Input: dimensioned drawing with shaded views. Units: mm. Origin: part minimum x, y, z. Give positions to 0.01 mm unless a question says otherwise; leave off trailing zeros. Loops run counter-clockwise (first coordinate to the right, second up) from the corner with the lowest first, then second, coordinate; pieces in that order, holes last. Notation, with made-up numbers: (-28, 18) -> (8, 18) arc R16 ccw to (8, 47) -> close; hole circle Ø3 at (57.5, 72). An arc over 180 degrees is marked (long way). Answer as a JSON object with one key per item and string values.
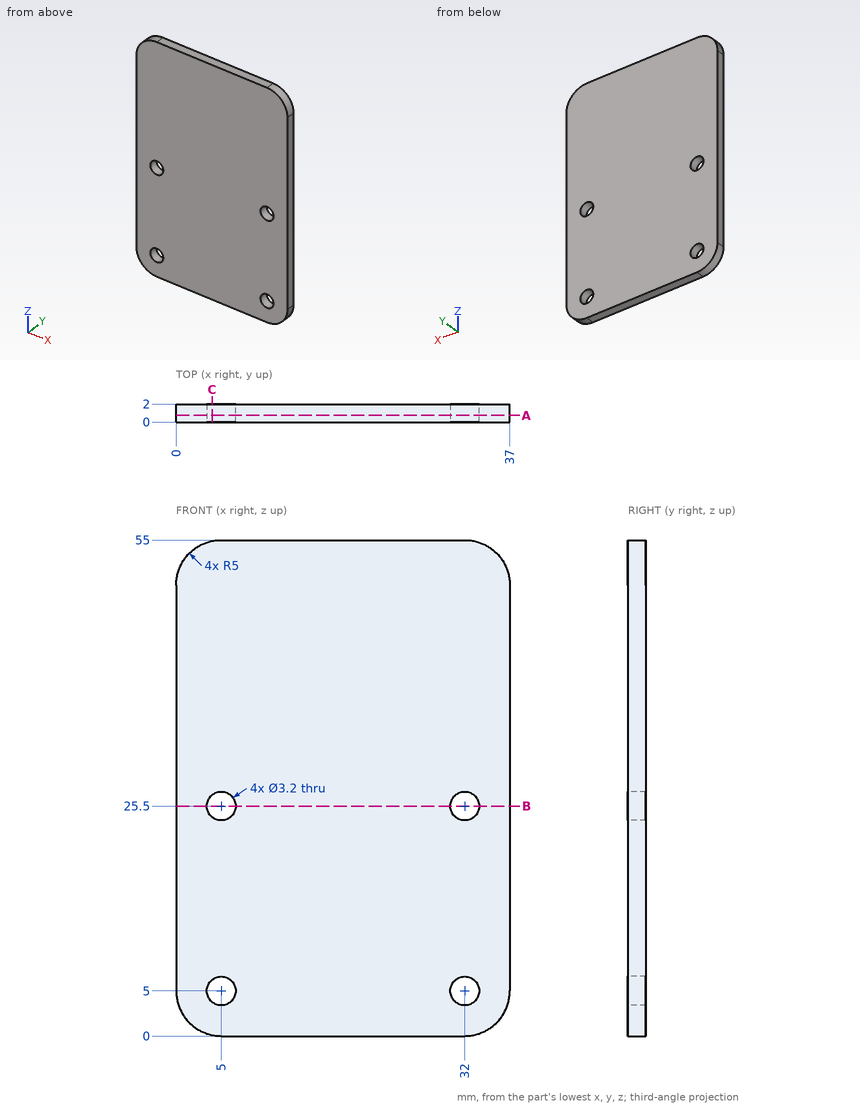
Q1. Ray query, line 1 along Z through (x, y) = (5, 0.8); line 2 along X through (y, z) = (0.9, 5); line 3 along X through (y, z) = (1.75, 4). Return the intervals inside material, ascending.
Evaluation:
{"line 1": "z = 0 to 3.4, 6.6 to 23.9, 27.1 to 55", "line 2": "x = 0 to 3.4, 6.6 to 30.4, 33.6 to 37", "line 3": "x = 0.1 to 3.75, 6.25 to 30.75, 33.25 to 36.9"}
Q2. Section B-B, the plane z = 25.5. Return the cut outline in (x, y).
Evaluation:
{"outline": "(0, 0) -> (3.4, 0) -> (3.4, 2) -> (0, 2) -> close; (6.6, 0) -> (30.4, 0) -> (30.4, 2) -> (6.6, 2) -> close; (33.6, 0) -> (37, 0) -> (37, 2) -> (33.6, 2) -> close"}
Q3. Section A-A, the plane y = 0.75. Return the cut outline in (x, z), then the cut area to 3 significant figures.
Evaluation:
{"outline": "(0, 5) arc R5 ccw to (5, 0) -> (32, 0) arc R5 ccw to (37, 5) -> (37, 50) arc R5 ccw to (32, 55) -> (5, 55) arc R5 ccw to (0, 50) -> close; hole circle Ø3.2 at (5, 5); hole circle Ø3.2 at (5, 25.5); hole circle Ø3.2 at (32, 5); hole circle Ø3.2 at (32, 25.5)", "area": "1,980 mm2"}
Q4. Section C-C, the plane x = 4. Return the cut outline in (y, z).
Evaluation:
{"outline": "(0, 0.1) -> (2, 0.1) -> (2, 3.75) -> (0, 3.75) -> close; (0, 6.25) -> (2, 6.25) -> (2, 24.25) -> (0, 24.25) -> close; (0, 26.75) -> (2, 26.75) -> (2, 54.9) -> (0, 54.9) -> close"}
